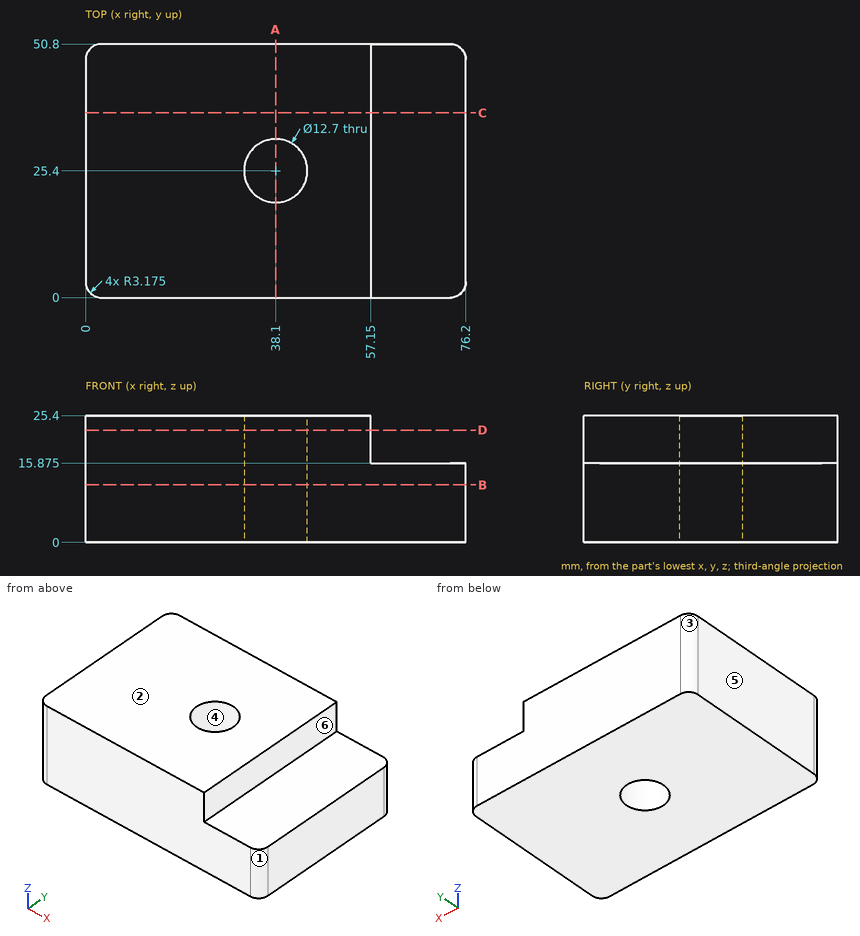
The drawing under review shows one solid part. Ordinate dimensions are in mm from its lowest x, y, z. A direction names the side the tool comes from. Round coordinates to 2 decimals unless told otherwise and drop trailing zeros. Write each loop counter-clockwise with the first axis right and the second up, starting at its lowest first coordinate (ties: lowest second). Pieces come first, ordered by that corner, then holes. Notation, with made-up numbers: (74, 11) - (110, 11) arc R33 ccw to (110, 41) - close; hole circle Ø2 at (13.25, -37.75). An arc over 180 degrees is marked (long way). Use a Markdown table: item, result. Add a question column.
1. We need section B-B (z = 11.5). State the section outline as (x, y) points (3 decimals), then the cut area to 3 significant figures.
2. We need section C-C (y = 37). State the section outline as (x, z) points (3 decimals).
3. Wall thickness on probe 1 along Y at (x, z) = (38.1, 14); probe 2 along X at (y, z) = (25, 10.75); probe 3 along X at (y, z) = (34, 18.75): over which ranges is each line inside the solid? List them lowest first.
4. Mouldability with a two-part tool opening along X and no side actions: class the marked faces 1, 2, 3 and 4 as +X half, -X half, draft (parallel to the pull), parting line (faces both ways), or undercut.
5. We need section A-A (x = 38.1). State the section outline as (y, z) points.
6. We need section D-D (z = 22.5). State the section outline as (x, y) points (3 decimals).
7. For the marked faces 5 and 6, list the 3-axis set-ups (+Z, -Z, +X, -X, +Y, -Y) from which the entire face can be reached by the end or side of a thin tool; tool diameter is ignored.
8. Clearance check with a flat-ended pin moving along its axis: pin 1 (21 mm diameter, centred on x = 64.5, y = 28.5, fed in from +Z). State where the tip first meets the part, or that it passes through.
Output:
| question | item | result |
|---|---|---|
| 1 | outline | (0, 3.175) arc R3.175 ccw to (3.175, 0) - (73.025, 0) arc R3.175 ccw to (76.2, 3.175) - (76.2, 47.625) arc R3.175 ccw to (73.025, 50.8) - (3.175, 50.8) arc R3.175 ccw to (0, 47.625) - close; hole circle Ø12.7 at (38.1, 25.4) |
| 1 | area | 3,740 mm2 |
| 2 | outline | (0, 0) - (76.2, 0) - (76.2, 15.875) - (57.15, 15.875) - (57.15, 25.4) - (0, 25.4) - close |
| 3 | probe 1 | y = 0 to 19.05, 31.75 to 50.8 |
| 3 | probe 2 | x = 0 to 31.76, 44.44 to 76.2 |
| 3 | probe 3 | x = 0 to 57.15 |
| 4 | face 1 | +X half |
| 4 | face 2 | draft |
| 4 | face 3 | -X half |
| 4 | face 4 | undercut |
| 5 | outline | (0, 0) - (19.05, 0) - (19.05, 25.4) - (0, 25.4) - close; (31.75, 0) - (50.8, 0) - (50.8, 25.4) - (31.75, 25.4) - close |
| 6 | outline | (0, 3.175) arc R3.175 ccw to (3.175, 0) - (57.15, 0) - (57.15, 50.8) - (3.175, 50.8) arc R3.175 ccw to (0, 47.625) - close; hole circle Ø12.7 at (38.1, 25.4) |
| 7 | face 5 | +Z, -Z, -X, +Y, -Y |
| 7 | face 6 | +Z, +X, +Y, -Y |
| 8 | pin 1 | stops at z = 25.4 |
